Answer from the drawing. Dimensions are ordinates in mm from the lowest x, y and z of the part. A direction names the side the tool comes from. Round coordinates to 2 decimals unless told otherwise and drop trailing zeros. Order: outer loops, then holes, each group sorted by start corner. A loop starts at its lowest first (then second) coordinate and runs counter-clockwise, first axis right, second up.
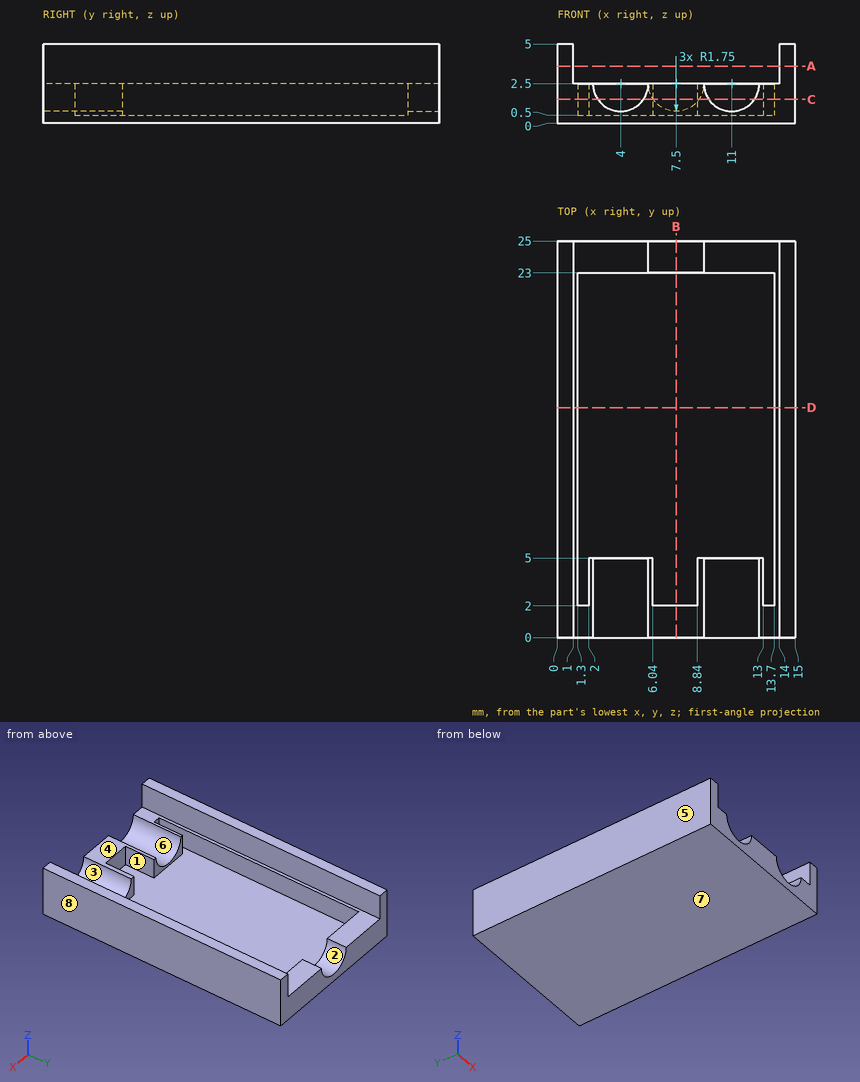
Q1. A cutting plane is placed at B-B, the plane x = 7.5. Give the vertices of the cut face in (y, z), plus the area to 3 significant figures.
Outcome:
outline: (0, 0) - (25, 0) - (25, 0.75) - (23, 0.75) - (23, 0.5) - (2, 0.5) - (2, 2.5) - (0, 2.5) - close
area: 17.0 mm2
Q2. A cutting plane is placed at A-A, the plane z = 3.6. Give the vertices of the cut face in (x, y), plus the area to 3 significant figures.
Outcome:
outline: (0, 0) - (1, 0) - (1, 25) - (0, 25) - close; (14, 0) - (15, 0) - (15, 25) - (14, 25) - close
area: 50.0 mm2
Q3. A cutting plane is placed at D-D, the plane y = 14.5. Give the vertices of the cut face in (x, z), plus the area to 3 significant figures.
Outcome:
outline: (0, 0) - (15, 0) - (15, 5) - (14, 5) - (14, 2.5) - (13.7, 2.5) - (13.7, 0.5) - (1.3, 0.5) - (1.3, 2.5) - (1, 2.5) - (1, 5) - (0, 5) - close
area: 17.7 mm2
Q4. For the marked faces 1, 2, 3 and 4, determine the directions among +Z, -Z, +X, -X, +Y, -Y from which every point of the face is accessible in a straight line to the end or side of a thin tool.
Outcome:
face 1: +Z
face 2: +Z, +Y
face 3: +Z, -Y
face 4: +Z, +Y, -Y
Q5. For a pull along X with two mould halves and no side action, classify the marked faces 5, 6, 7 and 8 as released by +X, released by -X, zero draft, split by the parting line, or undercut.
Outcome:
face 5: released by -X
face 6: undercut
face 7: zero draft
face 8: released by +X
Q6. Straight lines are drawn through the part: probe 1 along X at (y, z) = (13.75, 0.7); probe 2 along X at (y, z) = (7, 3.45); probe 3 along Y at (x, z) = (5.75, 1.9). For each, find the intervals that lie inside material, in ascending order.
Outcome:
probe 1: x = 0 to 1.3, 13.7 to 15
probe 2: x = 0 to 1, 14 to 15
probe 3: y = 0 to 5, 23 to 25
Q7. A cutting plane is placed at C-C, the plane z = 1.5. Give the vertices of the cut face in (x, y), plus the area to 3 significant figures.
Outcome:
outline: (0, 0) - (2.56, 0) - (2.56, 5) - (2, 5) - (2, 2) - (1.3, 2) - (1.3, 23) - (6.06, 23) - (6.06, 25) - (0, 25) - close; (5.44, 0) - (9.56, 0) - (9.56, 5) - (8.84, 5) - (8.84, 2) - (6.04, 2) - (6.04, 5) - (5.44, 5) - close; (8.94, 23) - (13.7, 23) - (13.7, 2) - (13, 2) - (13, 5) - (12.44, 5) - (12.44, 0) - (15, 0) - (15, 25) - (8.94, 25) - close
area: 105 mm2
Q8. A flat-ended cylindrical pin translates along its axis: pin 1 (1.4 mm diameter, centred on x = 3, y = 9.5, fed in from +Z). Find the tip coordinate at first contact, or state that the pin passes through.
Outcome:
pin 1: stops at z = 0.5
